Geometry check sheet. Reference: the model listing, model coordinates, mm. Face numbers are marked on the shaded views. A direction names the side the tool comes from. Round coordinates to 2 decimals unless told otherwise and drop trailing zeros. Loops run counter-clockwise (first coordinate to the right, second up) from the corner with the lowest first, then second, coordinate; pieces in that order, holes last.
```python
from build123d import *

# Parameters (mm, degrees)
F1_DEPTH        = 63.5
F2_DEPTH        = 15.875
F3_DEPTH        = 63.5
F0_W            = 19.05
F0_H            = 17.5050515682
F4_DEPTH        = 25.4
F5_DEPTH        = 25.4
F6_DEPTH        = 25.4
F7_DEPTH        = 12.7
F10_D           = 12.7
F10_ON_F0_D     = 12.7
F10_ON_F0_DEPTH = 63.501


with BuildPart() as f1:
    # F0 (on Front) → F1 (new body)
    with BuildSketch(Plane.XZ):
        Polygon((-36.0317155719, 0), (-36.0317155719, -19.05), (52.8682844281, -19.05), (52.8682844281, 0), (33.8182844281, 0), align=None)
    extrude(amount=F1_DEPTH)

    # F0 (on Front) → F2 (join)
    with BuildSketch(Plane.XZ):
        with BuildLine():
            ThreePointArc((50.590518862, 48.9809869127), (0.8347438774, 35.8877863894), (-36.0317155719, 0))
            Line((-36.0317155719, 0), (33.8182844281, 0))
            Line((33.8182844281, 0), (33.8182844281, 17.5050515682))
            Line((33.8182844281, 17.5050515682), (33.8182844281, 25.9368028492))
            ThreePointArc((33.8182844281, 25.9368028492), (38.4552849671, 40.1876121864), (50.590518862, 48.9809869127))
        make_face()
    extrude(amount=F2_DEPTH)

    # F0 (on Front) → F3 (join)
    with BuildSketch(Plane.XZ):
        Polygon((-36.0317155719, 0), (-36.0317155719, -19.05), (52.8682844281, -19.05), (52.8682844281, 0), (33.8182844281, 0), align=None)
    extrude(amount=-F3_DEPTH)

    # F0 (on Front) → F4 (join)
    with BuildSketch(Plane.XZ):
        with BuildLine():
            Line((60.4371747272, 48.9809869127), (50.590518862, 48.9809869127))
            ThreePointArc((50.590518862, 48.9809869127), (38.4552849671, 40.1876121864), (33.8182844281, 25.9368028492))
            Line((33.8182844281, 25.9368028492), (33.8182844281, 17.5050515682))
            Line((33.8182844281, 17.5050515682), (52.8682844281, 17.5050515682))
            Line((52.8682844281, 17.5050515682), (52.8682844281, 26.1928199722))
            ThreePointArc((52.8682844281, 26.1928199722), (54.9646325027, 31.2538519254), (60.0256644559, 33.3502))
            Line((60.0256644559, 33.3502), (60.6846340656, 33.3502))
            Line((60.6846340656, 33.3502), (60.6846340656, 48.9809869127))
            Line((60.6846340656, 48.9809869127), (60.4371747272, 48.9809869127))
        make_face()
        with Locations((43.3432844281, 8.7525257841)):
            Rectangle(F0_W, F0_H)
    extrude(amount=F4_DEPTH)

    # F0 (on Front) → F5 (join)
    with BuildSketch(Plane.XZ):
        with BuildLine():
            Line((60.4371747272, 48.9809869127), (50.590518862, 48.9809869127))
            ThreePointArc((50.590518862, 48.9809869127), (38.4552849671, 40.1876121864), (33.8182844281, 25.9368028492))
            Line((33.8182844281, 25.9368028492), (33.8182844281, 17.5050515682))
            Line((33.8182844281, 17.5050515682), (52.8682844281, 17.5050515682))
            Line((52.8682844281, 17.5050515682), (52.8682844281, 26.1928199722))
            ThreePointArc((52.8682844281, 26.1928199722), (54.9646325027, 31.2538519254), (60.0256644559, 33.3502))
            Line((60.0256644559, 33.3502), (60.6846340656, 33.3502))
            Line((60.6846340656, 33.3502), (60.6846340656, 48.9809869127))
            Line((60.6846340656, 48.9809869127), (60.4371747272, 48.9809869127))
        make_face()
        with Locations((43.3432844281, 8.7525257841)):
            Rectangle(F0_W, F0_H)
    extrude(amount=-F5_DEPTH)

    # F0 (on Front) → F6 (join)
    with BuildSketch(Plane.XZ):
        with Locations((43.3432844281, 8.7525257841)):
            Rectangle(F0_W, F0_H)
    extrude(amount=-F6_DEPTH)

    # F0 (on Front) → F7 (join)
    with BuildSketch(Plane.XZ):
        with BuildLine():
            ThreePointArc((50.590518862, 48.9809869127), (0.8347438774, 35.8877863894), (-36.0317155719, 0))
            Line((-36.0317155719, 0), (33.8182844281, 0))
            Line((33.8182844281, 0), (33.8182844281, 17.5050515682))
            Line((33.8182844281, 17.5050515682), (33.8182844281, 25.9368028492))
            ThreePointArc((33.8182844281, 25.9368028492), (38.4552849671, 40.1876121864), (50.590518862, 48.9809869127))
        make_face()
    extrude(amount=-F7_DEPTH)

    # F0 (on Front) → F8 (revolve)
    with BuildSketch(Plane.XZ):
        Polygon((60.6846340656, 53.8622255534), (60.6846340656, 48.9809869127), (60.6846340656, 33.3502), (60.8685202897, 33.3502), (60.8685202897, 25.2872255534), (86.0846340656, 25.2872255534), (86.0846340656, 53.8622255534), align=None)
    revolve(axis=Axis((60.6846340656, 0, 39.5747255534), (0, 0, -1)))

    # F10 (through all)
    with Locations(Plane.XY):
        with Locations((-13.4519258065, 50.5625051313), (34.9686927695, 50.6009981846), (31.0349383496, -49.7729142204), (-14.7181544946, -50.7195290418)):
            Hole(F10_D / 2)

    # F10 on F0 (through all, one way)
    with BuildSketch(Plane.XZ):
        with Locations((60.8685202897, 33.3502)):
            Circle(F10_ON_F0_D / 2)
    extrude(amount=-F10_ON_F0_DEPTH, mode=Mode.SUBTRACT)


solid = f1.part
```
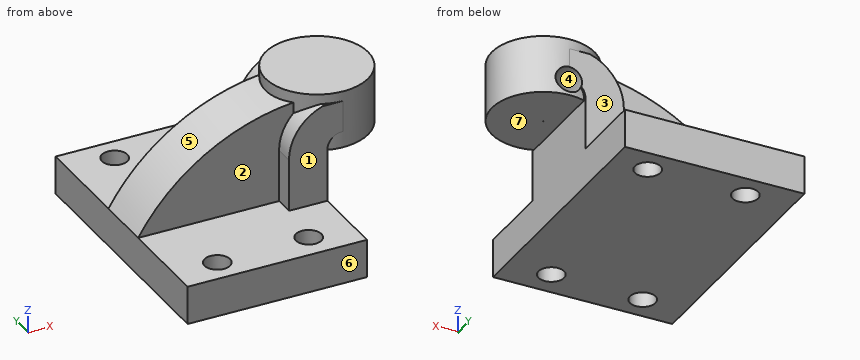
1) Mould release check, pull along Z, two halves, no side actions. Record for the marked faces 4, 5, 6 and 7: +Z half, -Z half, draft (parallel to the pull), parting line (faces both ways), or undercut.
Report:
face 4: undercut
face 5: +Z half
face 6: draft
face 7: -Z half
2) Access from +Z, -Z, +X, -X, +Y, -Y to the whole of each face (thin tool, end or side, straight path). Record for the marked faces 1, 2 and 3.
Report:
face 1: +Z, +X, -X, -Y
face 2: +Z, -X, -Y
face 3: +Z, +X, -X, +Y
3) Sectioned sample at D-D, the plane y = -36. Record the cut outline in (x, z), then the cut area to 3 significant figures.
Report:
outline: (-36.03, -19.05) - (52.87, -19.05) - (52.87, 0) - (-36.03, 0) - close
area: 1,690 mm2
4) Sectioned sample at A-A, the plane y = 17. Record the cut outline in (x, z).
Report:
outline: (-36.03, -19.05) - (52.87, -19.05) - (52.87, 25.29) - (79.56, 25.29) - (79.56, 53.86) - (41.81, 53.86) - (41.81, 43.92) arc R24.22 ccw to (33.82, 25.94) - (33.82, 0) - (-36.03, 0) - close; hole circle Ø12.7 at (60.87, 33.35)
5) Sectioned sample at B-B, the plane x = -14. Record the cut outline in (y, z) (3 decimals), then the cut area to 3 significant figures.
Report:
outline: (-63.5, -19.05) - (-57.029, -19.05) - (-57.029, 0) - (-63.5, 0) - close; (-44.41, -19.05) - (44.236, -19.05) - (44.236, 0) - (12.7, 0) - (12.7, 25.654) - (-15.875, 25.654) - (-15.875, 0) - (-44.41, 0) - close; (56.889, -19.05) - (63.5, -19.05) - (63.5, 0) - (56.889, 0) - close
area: 2,670 mm2
6) Sectioned sample at C-C, the plane z = 18. Record the cut outline in (x, y) (3 decimals).
Report:
outline: (-22.236, -15.875) - (33.818, -15.875) - (33.818, -25.4) - (52.868, -25.4) - (52.868, 25.4) - (33.818, 25.4) - (33.818, 12.7) - (-22.236, 12.7) - close
7) Gauge pin test, flat ends, axial feed: pin 1 (21.5 mm diameter, centred on x = 48, z = 13, fed in from -Y); pin 2 (14 mm diameter, centred on x = 62.5, z = 30.5, fed in from +Y); pin 3 (2 mm diameter, centred on y = 19, z = 19, fed in from -X). Record the tip position at first contact, or that the pin passes through.
Report:
pin 1: stops at y = -25.4
pin 2: stops at y = 25.4
pin 3: stops at x = 33.82
8) Scan lines: line 1 along X through (y, z) = (-46, -15); line 2 along X through (y, z) = (51, -9.5); line 3 along Y through (x, z) = (38, 2.5). Record each from-to range of solid material in increasing order.
Report:
line 1: x = -36.03 to -18.97, -10.47 to 25.93, 36.14 to 52.87
line 2: x = -36.03 to -19.79, -7.12 to 28.63, 41.31 to 52.87
line 3: y = -25.4 to 25.4
